Model file for the job. Use its own axes, mm. Face numbers are marked on the shaded views. Coordinates: 2 decimals unless noted, no trailing zeros. Order: outer loops, then holes, each group sorted by start corner. A loop starts at its lowest first (then second) coordinate and runs counter-clockwise, first axis right, second up.
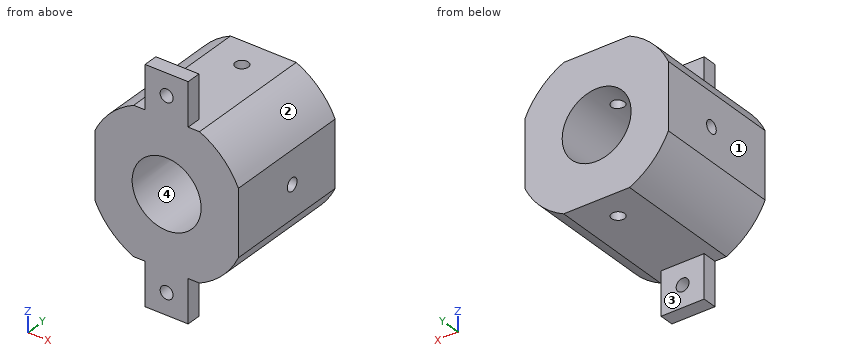
from build123d import *

# Parameters (mm, degrees)
BOSS_EXTRUDE1_DEPTH            = 45
SKETCH2_W                      = 15
SKETCH2_H                      = 5
BOSS_EXTRUDE2_DEPTH            = 15
SKETCH3_W                      = 15
SKETCH3_H                      = 5
BOSS_EXTRUDE3_DEPTH            = 15
F_24_0_24_DIAMETER_HOLE1_D     = 24
F_4_5_4_5_DIAMETER_HOLE1_D     = 4.5
F_4_5_4_5_DIAMETER_HOLE1_DEPTH = 63.212824766
F_4_5_4_5_DIAMETER_HOLE2_D     = 4.5
F_4_5_4_5_DIAMETER_HOLE2_DEPTH = 63.212824766
F_4_5_4_5_DIAMETER_HOLE3_D     = 4.5


with BuildPart() as part:
    # Sketch1 → Boss-Extrude1 (new body)
    with BuildSketch(Plane.XZ):
        with BuildLine():
            Line((-11.456439237, -25), (11.456439237, -25))
            ThreePointArc((11.456439237, -25), (19.445436483, -19.445436483), (25, -11.456439237))
            Line((25, -11.456439237), (25, 11.456439237))
            ThreePointArc((25, 11.456439237), (19.445436483, 19.445436483), (11.456439237, 25))
            Line((11.456439237, 25), (-11.456439237, 25))
            ThreePointArc((-11.456439237, 25), (-19.445436483, 19.445436483), (-25, 11.456439237))
            Line((-25, 11.456439237), (-25, -11.456439237))
            ThreePointArc((-25, -11.456439237), (-19.445436483, -19.445436483), (-11.456439237, -25))
        make_face()
    extrude(amount=-BOSS_EXTRUDE1_DEPTH)

    # Sketch2 → Boss-Extrude2 (add)
    with BuildSketch(Plane(origin=(0, 0, -25), x_dir=(-1, 0, 0), z_dir=(0, 0, -1))):
        with Locations((0, 2.5)):
            Rectangle(SKETCH2_W, SKETCH2_H)
    extrude(amount=BOSS_EXTRUDE2_DEPTH)

    # Sketch3 → Boss-Extrude3 (add)
    with BuildSketch(Plane.XY.offset(25)):
        with Locations((0, 2.5)):
            Rectangle(SKETCH3_W, SKETCH3_H)
    extrude(amount=BOSS_EXTRUDE3_DEPTH)

    # Ø24.0 (24) Diameter Hole1 (through all)
    with Locations(Plane(origin=(0, 0, 0), x_dir=(-1, 0, 0), z_dir=(0, -1, 0))):
        with Locations((0, 0)):
            Hole(F_24_0_24_DIAMETER_HOLE1_D / 2)

    # Ø4.5 (4.5) Diameter Hole1
    with Locations(Plane(origin=(0, 0, -25), x_dir=(-1, 0, 0), z_dir=(0, 0, -1))):
        with Locations((0, 35)):
            Hole(F_4_5_4_5_DIAMETER_HOLE1_D / 2, depth=F_4_5_4_5_DIAMETER_HOLE1_DEPTH)

    # Ø4.5 (4.5) Diameter Hole2
    with Locations(Plane.ZY.offset(25)):
        with Locations((0, 25)):
            Hole(F_4_5_4_5_DIAMETER_HOLE2_D / 2, depth=F_4_5_4_5_DIAMETER_HOLE2_DEPTH)

    # Ø4.5 (4.5) Diameter Hole3 (through all)
    with Locations(Plane(origin=(0, 5, 0), x_dir=(1, 0, 0), z_dir=(0, 1, 0))):
        with Locations((0, -32.5), (0, 32.5)):
            Hole(F_4_5_4_5_DIAMETER_HOLE3_D / 2)


solid = part.part
Q1. Mould opens along X. For the marked faces 1, 2, 3 and 4 say: pulls with the +X half, pulls with the -X half, needs draft (parallel to the pull), parting line crosses it, or undercut.
Established:
face 1: pulls with the -X half
face 2: pulls with the +X half
face 3: needs draft
face 4: undercut
Q2. Cut at D-D, the plane y = 20. List the corners of the cut face in (x, z), plus the area to 3 significant figures.
Established:
outline: (-25, -11.46) arc R27.5 ccw to (-11.46, -25) - (11.46, -25) arc R27.5 ccw to (25, -11.46) - (25, 11.46) arc R27.5 ccw to (11.46, 25) - (-11.46, 25) arc R27.5 ccw to (-25, 11.46) - close; hole circle Ø24 at (0, 0)
area: 1,770 mm2
Q3. Cut at A-A, the plane z = 32.5. List the corners of the cut face in (x, y), plus the area to 3 significant figures.
Established:
outline: (-7.5, 0) - (-2.25, 0) - (-2.25, 5) - (-7.5, 5) - close; (2.25, 0) - (7.5, 0) - (7.5, 5) - (2.25, 5) - close
area: 52.5 mm2
Q4. Drop flat-ended pins along their axis: P1, Ø3.5, axis at y = 25, z = 0, coming from the +X side; P2, Ø12, axis at x = 3, z = 32.5, coming from the +Y side; P3, Ø7, axis at x = 0, y = 35, coming from the +Z side; P4, Ø11.5, axis at x = 2, y = 28.5, coming from the -Z side. Give the stop position or say it passes through.
Established:
P1: passes through
P2: stops at y = 5
P3: stops at z = 25
P4: stops at z = -25
Q5. Cut at C-C, the plane x = 0. List the corners of the cut face in (y, z), plus the area to 3 significant figures.
Established:
outline: (0, -40) - (5, -40) - (5, -34.75) - (0, -34.75) - close; (0, -30.25) - (5, -30.25) - (5, -25) - (32.75, -25) - (32.75, -12) - (0, -12) - close; (0, 12) - (32.75, 12) - (32.75, 25) - (5, 25) - (5, 30.25) - (0, 30.25) - close; (0, 34.75) - (5, 34.75) - (5, 40) - (0, 40) - close; (37.25, -25) - (45, -25) - (45, -12) - (37.25, -12) - close; (37.25, 12) - (45, 12) - (45, 25) - (37.25, 25) - close
area: 1,160 mm2
Q6. Cut at B-B, the plane y = 25. List the corners of the cut face in (x, z).
Established:
outline: (-25, -11.46) arc R27.5 ccw to (-11.46, -25) - (11.46, -25) arc R27.5 ccw to (25, -11.46) - (25, -2.25) - (11.79, -2.25) arc R12 cw to (-11.79, -2.25) - (-25, -2.25) - close; (-25, 2.25) - (-11.79, 2.25) arc R12 cw to (11.79, 2.25) - (25, 2.25) - (25, 11.46) arc R27.5 ccw to (11.46, 25) - (-11.46, 25) arc R27.5 ccw to (-25, 11.46) - close
Q7. Probe line 1 (Z direction, x = 0, y = 1.7); line 2 (Y direction, x = -17.5, z = 0); line 3 (Z direction, x = 0, y = 14.5). List the from-to ranges inside material, lowest first.
Established:
line 1: z = -40 to -34.75, -30.25 to -12, 12 to 30.25, 34.75 to 40
line 2: y = 0 to 22.75, 27.25 to 45
line 3: z = -25 to -12, 12 to 25
